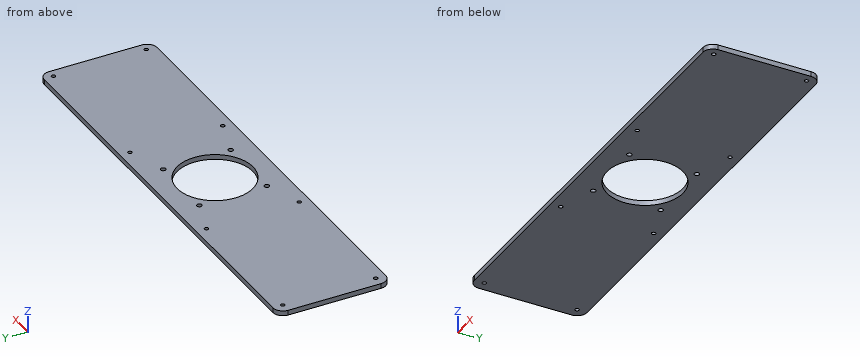
from build123d import *

# Parameters (mm, degrees)
ESQUISSE1_W        = 449
ESQUISSE1_H        = 113.5
ESQUISSE1_R        = 2
ESQUISSE1_R_2      = 38.25
ESQUISSE1_R_3      = 2.5
BOSS_EXTRU_1_DEPTH = 5
CONG_1_R           = 10


with BuildPart() as part:
    # Esquisse1 → Boss.-Extru.1 (new body)
    with BuildSketch(Plane.XY):
        with Locations((224.5, 56.75)):
            Rectangle(ESQUISSE1_W, ESQUISSE1_H)
        with Locations((10, 10)):
            Circle(ESQUISSE1_R, mode=Mode.SUBTRACT)
        with Locations((153.5, 10)):
            Circle(ESQUISSE1_R, mode=Mode.SUBTRACT)
        with Locations((297, 10)):
            Circle(ESQUISSE1_R, mode=Mode.SUBTRACT)
        with Locations((440.5, 10)):
            Circle(ESQUISSE1_R, mode=Mode.SUBTRACT)
        with Locations((153.5, 103.5)):
            Circle(ESQUISSE1_R, mode=Mode.SUBTRACT)
        with Locations((297, 103.5)):
            Circle(ESQUISSE1_R, mode=Mode.SUBTRACT)
        with Locations((440.5, 103.5)):
            Circle(ESQUISSE1_R, mode=Mode.SUBTRACT)
        with Locations((10, 103.5)):
            Circle(ESQUISSE1_R, mode=Mode.SUBTRACT)
        with Locations((224.5, 56.75)):
            Circle(ESQUISSE1_R_2, mode=Mode.SUBTRACT)
        with Locations((258.441125497, 90.691125497)):
            Circle(ESQUISSE1_R_3, mode=Mode.SUBTRACT)
        with Locations((258.441125497, 22.808874503)):
            Circle(ESQUISSE1_R_3, mode=Mode.SUBTRACT)
        with Locations((190.558874503, 22.808874503)):
            Circle(ESQUISSE1_R_3, mode=Mode.SUBTRACT)
        with Locations((190.558874503, 90.691125497)):
            Circle(ESQUISSE1_R_3, mode=Mode.SUBTRACT)
    extrude(amount=BOSS_EXTRU_1_DEPTH)

    # Congé1
    cong_1_edges = [part.edges().sort_by_distance(p)[0] for p in [
        (0, 113.5, 2.5),
        (449, 113.5, 2.5),
        (449, 0, 2.5),
        (0, 0, 2.5),
    ]]
    fillet(cong_1_edges, radius=CONG_1_R)


solid = part.part
Here's how the part is built. I have some questions about the finished solid (model axes, mm). Coordinates: 2 decimals unless noted, no trailing zeros. Write each loop counter-clockwise with the first axis right and the second up, starting at its lowest first coordinate (ties: lowest second). Pieces come first, ordered by that corner, then holes.
1) If we section it at A-A (y = 56.75): List the corners of the cut face in (x, z) for me, plus the area to 3 significant figures.
Filled in:
outline: (0, 0) - (186.25, 0) - (186.25, 5) - (0, 5) - close; (262.75, 0) - (449, 0) - (449, 5) - (262.75, 5) - close
area: 1,860 mm2
2) If I drill on line 1 (Y direction, x = 10, z = 3.8); line 2 (Y direction, x = 440.5, z = 3.1); line 3 (Y direction, x = 224.5, z = 2.35), over which ranges is the centre line in solid material (lowest first)?
Filled in:
line 1: y = 0 to 8, 12 to 101.5, 105.5 to 113.5
line 2: y = 0.11 to 8, 12 to 101.5, 105.5 to 113.39
line 3: y = 0 to 18.5, 95 to 113.5
3) If we section it at B-B (x = 224.5): List the corners of the cut face in (y, z) for me.
Filled in:
outline: (0, 0) - (18.5, 0) - (18.5, 5) - (0, 5) - close; (95, 0) - (113.5, 0) - (113.5, 5) - (95, 5) - close
4) If we section it at C-C (z = 1): Count the separate pieces of the cut face and the enclosed holes in it, plus the area to 3 significant figures.
Filled in:
separate pieces: 1
enclosed holes: 13
area: 46,100 mm2
5) I'm going to push flat-ended pins straight in: pin 1 (4 mm diameter, centred on x = 258.44, y = 90.69, fed in from -Z); pin 2 (5 mm diameter, centred on x = 321, y = 33.5, fed in from -Z). Where does each tip first touch, or does it pass through?
Filled in:
pin 1: passes through
pin 2: stops at z = 0
